Geometry check sheet. Reference: the model listing, model coordinates, mm. A direction names the side the tool comes from. Give positions to 0.01 mm unless a question says otherwise; leave off trailing zeros. Write each loop counter-clockwise with the first axis right and the second up, starting at its lowest first coordinate (ties: lowest second). Pieces come first, ordered by that corner, then holes. Notation, with made-up numbers: (8, 20) - (64, 20) arc R9 cw to (64, 24) - close; hole circle Ø3 at (35.25, 62.5). An arc over 180 degrees is marked (long way). Write item = value, one per line. Start each with the question number.
(1) Draft check along X on faces 1 (the flat face through (17.4, 17.5, 1.5)), 2 (the flat face through (28.186, 12.644, 1.479)), 3 (the flat face through (56.79, 17.09, 1.48)). Enter one of: pulls with the +X half, pulls with the -X half, needs draft (parallel to the pull), parting line crosses it, or undercut.
(2) Access from +Z, -Z, +X, -X, +Y, -Y to the whole of each face (thin tool, end or side, straight path). Record for faces 4 (the flat face through (33, -5, 1)), 5 (the flat face through (47.096, 12.861, 1.479)).
(3) Section check B-B, the plane x = 35. Enter the section's corners in (y, z), plus the area to 3 significant figures.
(4) Thickness scan on L1, parallel to Y at x = 49.5, z = 2.8; L2, parallel to Y at x = 20, z = 0.6; L3, parallel to X at y = -1, z = 1.9. Record the ranges inside material, lowest first.
(5) Section check A-A, the plane y = 0. Enter the section's corners in (x, z).
(6) Section check D-D, the plane y = 7. Enter the section's corners in (x, z).
(7) Depth check by flat-ended pin: pin 1 Ø2.5 at (x, y) = (40.87, 27.03) entering from -Z. Enter the tip coordinate at first touch or a pass-through.
(8) Section check C-C, the plane z = 1.4. Enter the section's corners in (x, y).
```python
from build123d import *

# Parameters (mm, degrees)
SKETCH1_R           = 1.5
BOSS_EXTRUDE1_DEPTH = 3


with BuildPart() as part:
    # Sketch1 → Boss-Extrude1 (new body)
    with BuildSketch(Plane.XY):
        with BuildLine():
            Line((-2.757874024, 4.170627155), (38.114272094, 31.197792594))
            ThreePointArc((38.114272094, 31.197792594), (41.479478747, 31.990143081), (44.554321247, 30.409706839))
            Line((44.554321247, 30.409706839), (69.382175128, 3.382541401))
            ThreePointArc((69.382175128, 3.382541401), (70.277810995, -2.01088202), (65.7, -5))
            Line((65.7, -5), (0, -5))
            ThreePointArc((0, -5), (-4.788169576, -1.439941705), (-2.757874024, 4.170627155))
        make_face()
        with Locations((40.872146119, 27.027165439)):
            Circle(SKETCH1_R, mode=Mode.SUBTRACT)
        Circle(SKETCH1_R, mode=Mode.SUBTRACT)
        with Locations((65.7, 0)):
            Circle(SKETCH1_R, mode=Mode.SUBTRACT)
        Polygon((40.074023256, 20.505095423), (54.317405325, 5), (16.626261885, 5), align=None, mode=Mode.SUBTRACT)
    extrude(amount=BOSS_EXTRUDE1_DEPTH)


solid = part.part
```
Model answer:
q1.face_1 = pulls with the -X half
q1.face_2 = undercut
q1.face_3 = pulls with the +X half
q2.face_4 = +Z, -Z, +X, -X, -Y
q2.face_5 = +Z, -Z
q3.outline = (-5, 0) - (5, 0) - (5, 3) - (-5, 3) - close; (17.15, 0) - (29.14, 0) - (29.14, 3) - (17.15, 3) - close
q3.area = 66.0 mm²
q4.L1 = -5 to 5, 10.24 to 25.03
q4.L2 = -5 to 5, 7.23 to 19.22
q4.L3 = -4.9 to -1.12, 1.12 to 64.58, 66.82 to 70.6
q5.outline = (-5, 0) - (-1.5, 0) - (-1.5, 3) - (-5, 3) - close; (1.5, 0) - (64.2, 0) - (64.2, 3) - (1.5, 3) - close; (67.2, 0) - (70.7, 0) - (70.7, 3) - (67.2, 3) - close
q6.outline = (1.52, 0) - (19.65, 0) - (19.65, 3) - (1.52, 3) - close; (52.48, 0) - (66.06, 0) - (66.06, 3) - (52.48, 3) - close
q7.pin_1 = through
q8.outline = (-2.76, 4.17) arc R5 ccw to (0, -5) - (65.7, -5) arc R5 ccw to (69.38, 3.38) - (44.55, 30.41) arc R5 ccw to (38.11, 31.2) - close; hole circle Ø3 at (0, 0); hole (16.63, 5) - (54.32, 5) - (40.07, 20.51) - close; hole circle Ø3 at (40.87, 27.03); hole circle Ø3 at (65.7, 0)
